The model under review builds one solid part; all positions refer to its coordinate system, in mm. Face numbers are marked on the shaded views. Coordinates: 2 decimals unless noted, no trailing zeros. Write each loop counter-clockwise with the first axis right and the second up, starting at its lowest first coordinate (ties: lowest second). Pieces come first, ordered by that corner, then holes. Notation, with made-up numbers: (-17.75, -7.5) - (-1.75, -7.5) arc R25 cw to (-1.75, 24.5) - close; hole circle Ø10 at (-23.75, 10). An arc over 180 degrees is marked (long way). Return JSON: item names as keys, results as strings. Group by question number.
(1) For pin 1 Ø1.5 at (x, z) = (-36, 28) entering from +Y; pin 2 Ø2.5 at (x, y) = (2.5, 9.5) entering from -Z; pin 3 Ø19.5 at (x, z) = (-59.5, 1) entering from +Y, all flat-tipped, find the tip position at first contact; note any pin that passes through.
(2) We need section C-C on y = 19.75. State the section outline as (x, z) points, then the cut area to 3 significant figures.
(3) We need section B-B on z = -37.5. State the section outline as (x, y) points.
(4) We need section A-A on x = 27.5. State the section outline as (y, z) points.
(5) Draft analysis for pull direction X (two halves, no side actions). For the marked faces 1, 2 and 3, state which applies: released by +X, released by -X, zero draft, split by the parting line, or undercut.
(6) To check wall thickness, follow L1, parallel to X at y = 10.75, z = 29; L2, parallel to X at y = 11.45, z = -10.16; L3, parallel to Y at x = 36, z = 29.5. State the ranges of each line that lie inside material, in increasing order. Write a range as from..to.
(7) We need section D-D on z = -67. State the section outline as (x, y) points, then the cut area to 3 significant figures.
```python
from build123d import *

# Parameters (mm, degrees)
SKETCH1_R           = 86.36
SKETCH1_R_2         = 83.82
BOSS_EXTRUDE1_DEPTH = 28.45
BOSS_EXTRUDE2_START = -1.27
SKETCH1_2_R         = 86.36
BOSS_EXTRUDE2_DEPTH = 1.27
SKETCH2_R           = 83.82
SKETCH2_R_2         = 2.413
BOSS_EXTRUDE3_DEPTH = 12.7
SKETCH3_R           = 1.651
SKETCH3_R_2         = 1.681286521
CUT_EXTRUDE1_DEPTH  = 2.54
CUT_EXTRUDE2_START  = -7.62
CUT_EXTRUDE2_DEPTH  = 7.62


with BuildPart() as part:
    # Sketch1 → Boss-Extrude1 (new body)
    with BuildSketch(Plane(origin=(0, 0, 0), x_dir=(1, 0, 0), z_dir=(0, 1, 0))):
        with Locations(Location((0, 0, 0), (0, 0, 270))):
            Circle(SKETCH1_R)
        with Locations(Location((0, 0, 0), (0, 0, 270))):
            Circle(SKETCH1_R_2, mode=Mode.SUBTRACT)
    extrude(amount=BOSS_EXTRUDE1_DEPTH)

    # Sketch1_2 → Boss-Extrude2 (add)
    with BuildSketch(Plane(origin=(0, 0, 0), x_dir=(1, 0, 0), z_dir=(0, 1, 0)).offset(BOSS_EXTRUDE2_START)):
        with Locations(Location((0, 0, 0), (0, 0, 270))):
            Circle(SKETCH1_2_R)
    extrude(amount=BOSS_EXTRUDE2_DEPTH)

    # Sketch2 → Boss-Extrude3 (add)
    with BuildSketch(Plane(origin=(0, 0, 0), x_dir=(1, 0, 0), z_dir=(0, 1, 0))):
        with Locations(Location((0, 0, 0), (0, 0, 270))):
            Circle(SKETCH2_R)
        with Locations(Location((44.845, 44.845, 0), (0, 0, 270))):
            Circle(SKETCH2_R_2, mode=Mode.SUBTRACT)
        with Locations(Location((44.845, -44.845, 0), (0, 0, 270))):
            Circle(SKETCH2_R_2, mode=Mode.SUBTRACT)
        with Locations(Location((-44.845, -44.845, 0), (0, 0, 270))):
            Circle(SKETCH2_R_2, mode=Mode.SUBTRACT)
        with Locations(Location((-44.845, 44.845, 0), (0, 0, 270))):
            Circle(SKETCH2_R_2, mode=Mode.SUBTRACT)
    extrude(amount=BOSS_EXTRUDE3_DEPTH)

    # Sketch3 → Cut-Extrude1 (cut)
    with BuildSketch(Plane(origin=(0, 12.7, 0), x_dir=(1, 0, 0), z_dir=(0, 1, 0))):
        with Locations(Location((6.35, 10.16, 0), (0, 0, 270))):
            Circle(SKETCH3_R)
        with Locations(Location((6.35, -10.16, 0), (0, 0, 270))):
            Circle(SKETCH3_R)
        with Locations(Location((-6.35, -10.16, 0), (0, 0, 270))):
            Circle(SKETCH3_R)
        with Locations(Location((-6.35, 10.16, 0), (0, 0, 270))):
            Circle(SKETCH3_R_2)
    extrude(amount=-CUT_EXTRUDE1_DEPTH, mode=Mode.SUBTRACT)

    # Sketch4 → Cut-Extrude2 (cut)
    with BuildSketch(Plane(origin=(0, 12.7, 0), x_dir=(1, 0, 0), z_dir=(0, 1, 0)).offset(CUT_EXTRUDE2_START)):
        with BuildLine():
            Line((-70.12180118, 45.920860176), (-19.05, 10.16))
            Line((-19.05, 10.16), (-19.05, -10.16))
            Line((-19.05, -10.16), (-70.12180118, -45.920860176))
            ThreePointArc((-70.12180118, -45.920860176), (-83.82, 0), (-70.12180118, 45.920860176))
        make_face()
        with BuildLine():
            Line((-10.16, 19.05), (10.16, 19.05))
            Line((10.16, 19.05), (45.920860176, 70.12180118))
            ThreePointArc((45.920860176, 70.12180118), (0, 83.82), (-45.920860176, 70.12180118))
            Line((-45.920860176, 70.12180118), (-10.16, 19.05))
        make_face()
        with BuildLine():
            Line((19.05, 10.16), (19.05, -10.16))
            Line((19.05, -10.16), (70.12180118, -45.920860176))
            ThreePointArc((70.12180118, -45.920860176), (83.82, 0), (70.12180118, 45.920860176))
            Line((70.12180118, 45.920860176), (19.05, 10.16))
        make_face()
        with BuildLine():
            Line((10.16, -19.05), (-10.16, -19.05))
            Line((-10.16, -19.05), (-45.920860176, -70.12180118))
            ThreePointArc((-45.920860176, -70.12180118), (0, -83.82), (45.920860176, -70.12180118))
            Line((45.920860176, -70.12180118), (10.16, -19.05))
        make_face()
    extrude(amount=CUT_EXTRUDE2_DEPTH, mode=Mode.SUBTRACT)


solid = part.part
```
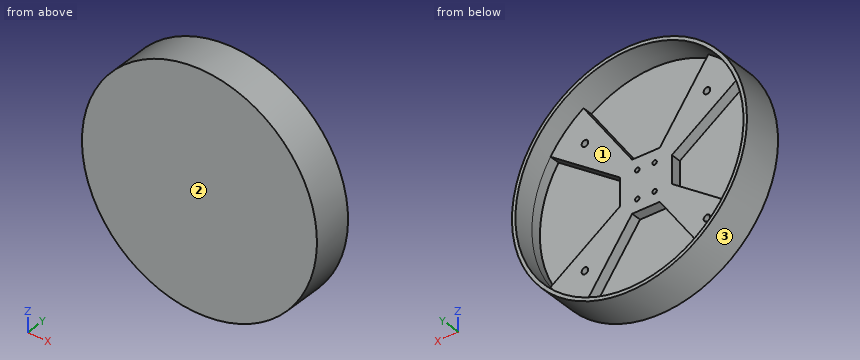
Ans:
{
 "1": {"pin 1": "y = 12.7", "pin 2": "z = -86.35", "pin 3": "y = 5.08"},
 "2": {"outline": "circle Ø172.72 at (0, 0); hole circle Ø167.64 at (0, 0)", "area": "1,360 mm²"},
 "3": {"outline": "(-77.79, -1.27) - (77.79, -1.27) - (77.79, 28.45) - (74.96, 28.45) - (74.96, 5.08) - (58.1, 5.08) - (58.1, 12.7) - (23.08, 12.7) - (23.08, 5.08) - (-23.08, 5.08) - (-23.08, 12.7) - (-58.1, 12.7) - (-58.1, 5.08) - (-74.96, 5.08) - (-74.96, 28.45) - (-77.79, 28.45) - close"},
 "4": {"outline": "(-1.27, -81.86) - (28.45, -81.86) - (28.45, -79.18) - (5.08, -79.18) - (5.08, -43.81) - (12.7, -43.81) - (12.7, -16.08) - (5.08, -16.08) - (5.08, 16.08) - (12.7, 16.08) - (12.7, 43.81) - (5.08, 43.81) - (5.08, 79.18) - (28.45, 79.18) - (28.45, 81.86) - (-1.27, 81.86) - close"},
 "5": {"face 1": "undercut", "face 2": "zero draft", "face 3": "split by the parting line"},
 "6": {"L1": "-81.35..-78.64, -45.96..-17.13, 17.13..45.96, 78.64..81.35", "L2": "-85.76..-83.2, -19.05..-8.03, -4.67..4.7, 8..19.05, 83.2..85.76", "L3": "-1.27..12.7"},
 "7": {"outline": "(-54.49, -1.27) - (54.49, -1.27) - (54.49, 28.45) - (50.37, 28.45) - (50.37, 12.7) - (43.73, 12.7) - (43.73, 5.08) - (-43.73, 5.08) - (-43.73, 12.7) - (-50.37, 12.7) - (-50.37, 28.45) - (-54.49, 28.45) - close", "area": "986 mm²"}
}
